Verification items for the finished model (mm, model axes). A direction names the side the tool comes from. Round coordinates to 2 decimals unless told otherwise and drop trailing zeros. Loops run counter-clockwise (first coordinate to the right, second up) from the corner with the lowest first, then second, coordinate; pieces in that order, holes last. Notation, with made-up numbers: (-23.75, -21.5) -> (19.25, -21.5) arc R17 ccw to (19.25, -3.5) -> close; hole circle Ø8 at (-26.5, -13.5). An arc over 180 degrees is marked (long way). Use CSV: the item, a comma, the result in double quotes. Start each with the question number.
```python
from build123d import *

# Parameters (mm, degrees)
BOSS_EXTRUDE1_DEPTH = 15
BOSS_EXTRUDE3_DEPTH = 10


with BuildPart() as part:
    # Sketch1 → Boss-Extrude1 (new body, symmetric)
    with BuildSketch(Plane.XY):
        with BuildLine():
            Line((-22, 110), (-22, 82))
            ThreePointArc((-22, 82), (0, 60), (22, 82))
            Line((22, 82), (22, 110))
            ThreePointArc((22, 110), (0, 132), (-22, 110))
        make_face()
        with BuildLine():
            Line((10, 110), (10, 97.763084363))
            ThreePointArc((10, 97.763084363), (11.449489743, 96.666708046), (12, 94.934657238))
            Line((12, 94.934657238), (12, 82))
            ThreePointArc((12, 82), (0, 70), (-12, 82))
            Line((-12, 82), (-12, 94.322221654))
            ThreePointArc((-12, 94.322221654), (-11.449489743, 96.054272461), (-10, 97.150648779))
            Line((-10, 97.150648779), (-10, 110))
            ThreePointArc((-10, 110), (0, 120), (10, 110))
        make_face(mode=Mode.SUBTRACT)
    extrude(amount=BOSS_EXTRUDE1_DEPTH, both=True)

    # Sketch1_4 → Boss-Extrude3 (add, symmetric)
    with BuildSketch(Plane.XY):
        with BuildLine():
            ThreePointArc((20.54909502, 117.857142857), (21.634233178, 113.994991212), (22, 110))
            Line((22, 110), (22, 82))
            ThreePointArc((22, 82), (0, 60), (-22, 82))
            Line((-22, 82), (-22, 110))
            ThreePointArc((-22, 110), (-21.634233178, 113.994991212), (-20.54909502, 117.857142857))
            Line((-20.54909502, 117.857142857), (-29.889592756, 93.428571429))
            ThreePointArc((-29.889592756, 93.428571429), (-31.795758241, 78.390324411), (-26.567056796, 64.162077105))
            ThreePointArc((-26.567056796, 64.162077105), (-21.561800954, 45.141212789), (-29.413527167, 27.108013937))
            ThreePointArc((-29.413527167, 27.108013937), (0, -40), (29.413527167, 27.108013937))
            ThreePointArc((29.413527167, 27.108013937), (21.561800954, 45.141212789), (26.567056796, 64.162077105))
            ThreePointArc((26.567056796, 64.162077105), (31.795758241, 78.390324411), (29.889592756, 93.428571429))
            Line((29.889592756, 93.428571429), (20.54909502, 117.857142857))
        make_face()
        with BuildLine():
            Line((11.968538667, 9.131620953), (10, -18))
            ThreePointArc((10, -18), (0.357371137, -27.993612253), (-9.974457174, -18.714285714))
            Line((-9.974457174, -18.714285714), (-11.969348609, 9.142857143))
            ThreePointArc((-11.969348609, 9.142857143), (0.005632672, 21.999998678), (11.968538667, 9.131620953))
        make_face(mode=Mode.SUBTRACT)
    extrude(amount=BOSS_EXTRUDE3_DEPTH, both=True)


solid = part.part
```
Q1. Depth check by flat-ended pin: pin 1 Ø10.5 at (y, z) = (105.5, 4) entering from +X; pin 2 Ø4 at (y, z) = (62.5, 10) entering from +X; pin 3 Ø4 at (x, y) = (9.5, 6.5) entering from -Z; pin 4 Ø8 at (y, z) = (33.5, 10) entering from -X. Enter the tip coordinate at first touch or a pass-through.
Q2. Tool access check on faces 1 (the face through (-31.82, 78.6, 0.14)), 2 (the face through (22, 96, 13)), 3 (the face through (0, 22, 0)). Record the directions out of +Z, -Z, +X, -X, +Y, -Y that give a thin tool (end or side, any length) a straight path to the whole face; none if there is none.
Q3. Cross-section at B-B (x = 0). Record the boundary of the cut face in (y, z), and give its area (3 significant figures).
Q4. Cross-section at C-C (y = 13). Record the boundary of the cut face in (x, z), and give its area (3 significant figures).
Q5. Cross-section at D-D (z = -12.25). Record the boundary of the cut face in (x, y), and give its area (3 significant figures).
Q6. Release check for a two-part mould opening along Y. For faces 4 (the face through (0, 60, 13)), 5 (the face through (-10, 103, 0)), 6 (the face through (14, 97, 15)) record: +Y half, -Y half, draft (parallel to the pull), parting line (faces both ways), or undercut.
Q7. Thickness scan on L1, parallel to Y at x = -3, z = -9.75; L2, parallel to Z at x = -19, y = 14; L3, parallel to Y at x = -5.5, z = -1.75. Record the ranges inside material, lowest first. Write a range as from..to.
Q8. Cross-section at A-A (z = -1). Record the boundary of the cut face in (x, y).
Answer list:
1,pin 1,"stops at x = 27.28"
1,pin 2,"stops at x = 26.79"
1,pin 3,"passes through"
1,pin 4,"stops at x = -27.43"
2,face 1,"+Z, -Z, -X"
2,face 2,"+Z, +X, +Y, -Y"
2,face 3,"+Z, -Z"
3,outline,"(-40, -10) -> (-28, -10) -> (-28, 10) -> (-40, 10) -> close; (22, -10) -> (60, -10) -> (60, -15) -> (70, -15) -> (70, 15) -> (60, 15) -> (60, 10) -> (22, 10) -> close; (120, -15) -> (132, -15) -> (132, 15) -> (120, 15) -> close"
3,area,"1,660 mm2"
4,outline,"(-37.83, -10) -> (-11.62, -10) -> (-11.62, 10) -> (-37.83, 10) -> close; (11.62, -10) -> (37.83, -10) -> (37.83, 10) -> (11.62, 10) -> close"
4,area,"1,050 mm2"
5,outline,"(-22, 82) arc R22 ccw to (22, 82) -> (22, 110) arc R22 ccw to (-22, 110) -> close; hole (-12, 82) arc R12 ccw to (12, 82) -> (12, 94.93) arc R3 ccw to (10, 97.76) -> (10, 110) arc R10 ccw to (-10, 110) -> (-10, 97.15) arc R3 ccw to (-12, 94.32) -> close"
5,area,"1,750 mm2"
6,face 4,"-Y half"
6,face 5,"undercut"
6,face 6,"draft"
7,L1,"y = -39.89..-27.54, 21.62..70.38, 119.54..131.79"
7,L2,"z = -10..10"
7,L3,"y = -39.62..-26.35, 20.67..71.33, 118.35..131.3"
8,outline,"(-29.89, 93.43) arc R32 ccw to (-26.57, 64.16) arc R30 cw to (-29.41, 27.11) arc R40 ccw (long way) to (29.41, 27.11) arc R30 cw to (26.57, 64.16) arc R32 ccw to (29.89, 93.43) -> (20.55, 117.86) arc R22 ccw to (-20.55, 117.86) -> close; hole (-12, 82) arc R12 ccw to (12, 82) -> (12, 94.93) arc R3 ccw to (10, 97.76) -> (10, 110) arc R10 ccw to (-10, 110) -> (-10, 97.15) arc R3 ccw to (-12, 94.32) -> close; hole (-11.97, 9.14) -> (-9.97, -18.71) arc R10 ccw to (10, -18) -> (11.97, 9.13) arc R12 ccw (long way) to start"
